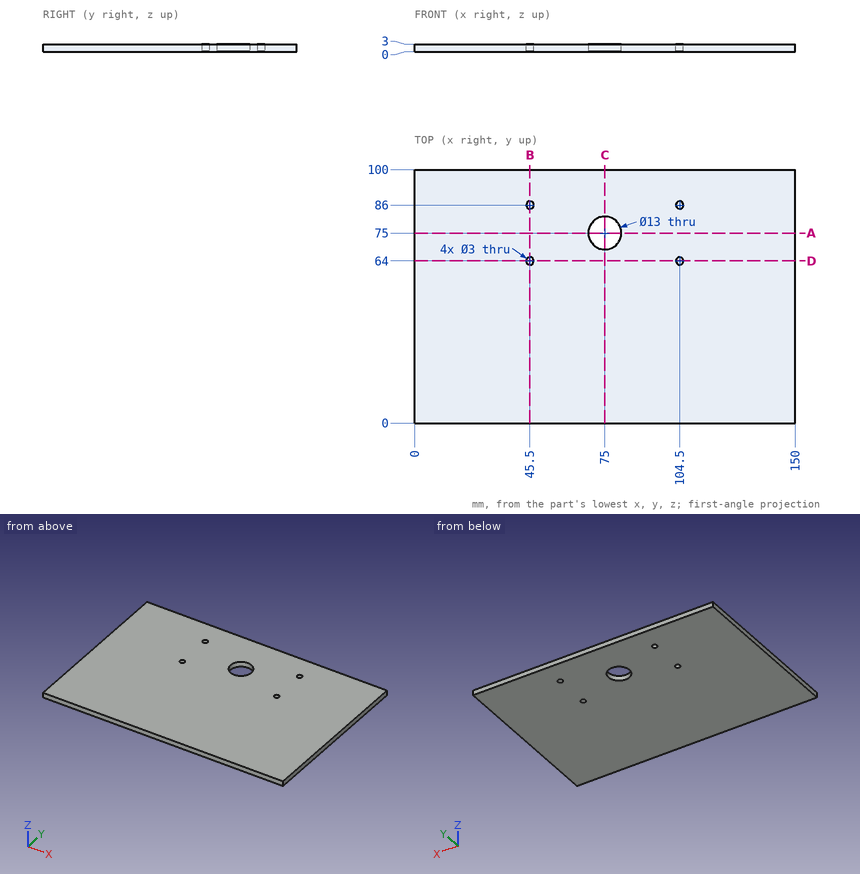
Could you check a few things on this drawing? It's one solid part, dimensions in mm from its lowest x, y, z. Give positions to 0.01 mm unless a question says otherwise; leave off trailing zeros. Loops run counter-clockwise (first coordinate to the right, second up) from the corner with the lowest first, then second, coordinate; pieces in that order, holes last. Notation, with made-up numbers: M 55,-24 L 59,-24 A20 ccw 59,-14 Z; hole C -36.75,79 d6. An arc over 180 degrees is marked long. One line per question, with ' | ' between items. Start each with the question number.
Q1. For pin 1 Ø3.5 at (x, y) = (104.5, 64) entering from +Z; pin 2 Ø2.5 at (x, y) = (104.5, 86) entering from -Z, each with a flat end and sliding along its axis, tell me the tip position at first contact or that it passes through.
Q2. If we section it at C-C (x = 75): Please give me the cut outline in (y, z), plus the area to 3 significant figures.
Q3. If we section it at D-D (y = 64): Please give me the cut outline in (x, z).
Q4. If we section it at A-A (y = 75): Please give me the cut outline in (x, z), plus the area to 3 significant figures.
Q5. If I drill on line 1 (X direction, y = 64, z = 1.05); line 2 (Y direction, x = 45.5, z = 0.75); line 3 (X direction, y = 63, z = 1.5), over which ranges is the centre line in solid material (lowest first)? Write a range as from..to.
Q6. If we section it at B-B (x = 45.5): Please give me the cut outline in (y, z).
Computed:
1) pin 1: stops at z = 3 | pin 2: passes through
2) outline: M 0,0 L 68.5,0 L 68.5,3 L 0,3 Z; M 81.5,0 L 100,0 L 100,3 L 81.5,3 Z | area: 261 mm²
3) outline: M 0,0 L 44,0 L 44,3 L 0,3 Z; M 47,0 L 103,0 L 103,3 L 47,3 Z; M 106,0 L 150,0 L 150,3 L 106,3 Z
4) outline: M 0,0 L 68.5,0 L 68.5,3 L 0,3 Z; M 81.5,0 L 150,0 L 150,3 L 81.5,3 Z | area: 411 mm²
5) line 1: x = 0..44, 47..103, 106..150 | line 2: y = 0..62.5, 65.5..84.5, 87.5..100 | line 3: x = 0..44.38, 46.62..103.38, 105.62..150
6) outline: M 0,0 L 62.5,0 L 62.5,3 L 0,3 Z; M 65.5,0 L 84.5,0 L 84.5,3 L 65.5,3 Z; M 87.5,0 L 100,0 L 100,3 L 87.5,3 Z
